Verification items for the finished model (mm, model axes). A direction names the side the tool comes from. Coordinates: 2 decimals unless noted, no trailing zeros. Order: outer loops, then holes, each group sorted by start corner. A loop starts at its lowest first (then second) coordinate and runs counter-clockwise, first axis right, second up. Notation, with made-up numbers: M 13,-15 L 27,-15 A17 cw 27,15 Z; hole C 89.25,-15 d6. An arc over 180 degrees is marked long. Answer as a JSON object with one key per item and string values. Group by question number.
(1) Mould release check, pull along Y, two halves, no side actions. Record for faces 1 (the face through (39.43, 24.4, 9.21)), 2 (the face through (-1, 0, 0)), 3 (the face through (-35.4, 29.2, 0.8)), 4 (the face through (39.4, -24.43, 9.21)): released by +Y, released by -Y, zero draft, split by the parting line, or undercut.
(2) Material ranges on line 1 (X direction, y = -31.75, z = 1); line 2 (Y direction, x = -11.5, z = 8.75); line 3 (X direction, y = 20.5, z = 3), recorded low to high.
(3) Gauge pin test, flat ends, axial feed: pin 1 Ø7.5 at (y, z) = (-11, 10) entering from +X; pin 2 Ø4 at (x, z) = (22, 8.5) entering from -Y; pin 3 Ø2 at (x, y) = (33, -26.75) entering from +Z. Record the tip position at first contact, or that the pin passes through.
(4) Cross-section at A-A (y = -9.5). Enter the section's corners in (x, z), plus the area to 3 significant figures.
(5) Access from +Z, -Z, +X, -X, +Y, -Y to the whole of each face (thin tool, end or side, straight path). Record for faces 5 (the face through (30.6, -29.3, 0.8)), 6 (the face through (-39.4, 24.43, 9.21)), 7 (the face through (1, 25, 9)).
(6) Cross-section at B-B (z = 11.25). Enter the section's corners in (x, y), plus the area to 3 significant figures.
Autodesk Inventor part; units mm, degrees
ref_plane "YZ Plane" through (0, 0, 0) normal (1, 0, 0) x (0, 1, 0)
ref_plane "XZ Plane" through (0, 0, 0) normal (0, 1, 0) x (-1, 0, 0)
ref_plane "XY Plane" through (0, 0, 0) normal (0, 0, 1) x (1, 0, 0)
sketch "Sketch1" plane through (0, 0, 0) normal (0, 0, 1) x (1, 0, 0)
  line L0 (41, 33.5) -> (-41, 33.5)
  line L1 (-41, 33.5) -> (-41, -33.5)
  line L2 (-41, -33.5) -> (41, -33.5)
  line L3 (41, -33.5) -> (41, 33.5)
  line L4 (41, 33.5) -> (-41, -33.5) construction
  line L5 (-41, 33.5) -> (41, -33.5) construction
  line L6 (-33, 29.25) -> (33, 29.25) construction
  line L7 (33, 29.25) -> (33, -29.25) construction
  line L8 (33, -29.25) -> (-33, -29.25) construction
  line L9 (-33, -29.25) -> (-33, 29.25) construction
  line L10 (-33, 29.25) -> (33, -29.25) construction
  line L11 (33, 29.25) -> (-33, -29.25) construction
  line L12 (41, 0) -> (-41, 0) construction
  line L13 (0, 33.5) -> (0, -33.5) construction
  circle A0 centre (33, 29.25) radius 2.4
  circle A1 centre (-33, 29.25) radius 2.4
  circle A2 centre (33, -29.25) radius 2.4
  circle A3 centre (-33, -29.25) radius 2.4
  line L14 (33, 32.5) -> (33, 26) construction
  arc A4 (32.2801, 26.9605) -> (33.7199, 26.9605) centre (33, 26.75) ccw
  arc A5 (-33.7199, 26.9605) -> (-32.2801, 26.9605) centre (-33, 26.75) ccw
  arc A6 (33.7199, -26.9605) -> (32.2801, -26.9605) centre (33, -26.75) ccw
  arc A7 (-32.2801, -26.9605) -> (-33.7199, -26.9605) centre (-33, -26.75) ccw
  line L15 (40, 25) -> (-40, 25)
  line L16 (-40, 25) -> (-40, -25)
  line L17 (-40, -25) -> (40, -25)
  line L18 (40, -25) -> (40, 25)
  line L19 (40, 25) -> (-40, -25) construction
  line L20 (-40, 25) -> (40, -25) construction
  arc A8 (33.7199, 31.5395) -> (32.2801, 31.5395) centre (33, 31.75) ccw
  arc A9 (-32.2801, 31.5395) -> (-33.7199, 31.5395) centre (-33, 31.75) ccw
  arc A10 (32.2801, -31.5395) -> (33.7199, -31.5395) centre (33, -31.75) ccw
  arc A11 (-33.7199, -31.5395) -> (-32.2801, -31.5395) centre (-33, -31.75) ccw
  point P0 (0, 0)
  point P1 (33, -26)
  point P2 (-32.2801, 26.9605)
  point P3 (-33.7199, 26.9605)
  point P4 (-33.7199, -26.9605)
  point P5 (-32.2801, -26.9605)
  point P6 (32.2801, -26.9605)
  point P7 (33.7199, -26.9605)
  point P8 (33, 32.5)
  point P9 (32.2801, 31.5395)
  point P10 (33.7199, 31.5395)
  point P11 (-33.7199, 31.5395)
  point P12 (-32.2801, 31.5395)
  point P13 (-32.2801, -31.5395)
  point P14 (-33.7199, -31.5395)
  point P15 (33.7199, -31.5395)
  point P16 (32.2801, -31.5395)
  dimension "d0" = 82
  dimension "d1" = 67
  dimension "d19" = 4.8
  dimension "d30" = 6.5
  dimension "d33" = 58.5
  dimension "d34" = 66
  dimension "d36" = 1.5
  dimension "d37" = 8.5
  dimension "d38" = 1
  dimension "d41" = 16
  dimension "d42" = 6.5
  dimension "d43" = 1
extrude "Extrusion1" add sketch "Sketch1" along normal blind 1.6 contours L3 L2 L1 L0 | L18 L17 L16 L15
extrude "Extrusion2" add sketch "Sketch1" along normal blind 16.6 contours L18 L17 L16 L15
fillet "Fillet1" radius 2 4 edges at (40, -25, 9.1) (40, 25, 9.1) (-40, -25, 9.1) (-40, 25, 9.1)
properties part number "SUSTAINA-ACTUATOR-POWER-BOARD" material "Acetal Resin, Black"
Taken from the geometry:
{
 "1": {"face 1": "released by +Y", "face 2": "zero draft", "face 3": "undercut", "face 4": "released by -Y"},
 "2": {"line 1": "x = -41 to -33.75, -32.25 to 32.25, 33.75 to 41", "line 2": "y = -25 to 25", "line 3": "x = -40 to 40"},
 "3": {"pin 1": "stops at x = 40", "pin 2": "stops at y = -25", "pin 3": "stops at z = 1.6"},
 "4": {"outline": "M -41,0 L 41,0 L 41,1.6 L 40,1.6 L 40,16.6 L -40,16.6 L -40,1.6 L -41,1.6 Z", "area": "1,330 mm²"},
 "5": {"face 5": "+Z, -Z", "face 6": "+Z, -X, +Y", "face 7": "+Z, +X, -X, +Y"},
 "6": {"outline": "M -40,-23 A2 ccw -38,-25 L 38,-25 A2 ccw 40,-23 L 40,23 A2 ccw 38,25 L -38,25 A2 ccw -40,23 Z", "area": "4,000 mm²"}
}
